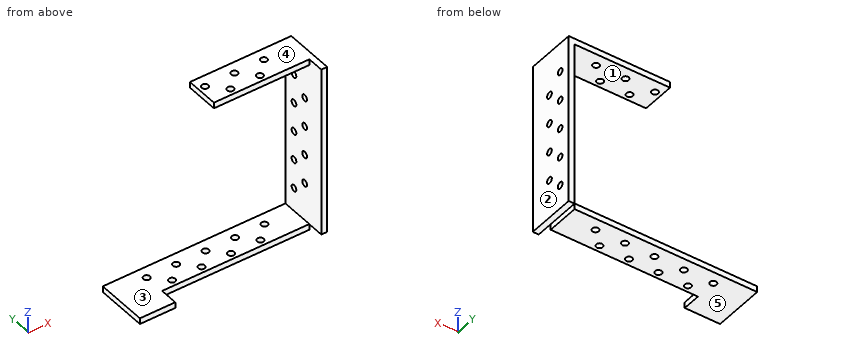
```python
from build123d import *

# Parameters (mm, degrees)
SKETCH1_W                      = 42
SKETCH1_H                      = 145.161285219
BOSS_EXTRUDE1_DEPTH            = 5
BOSS_EXTRUDE2_DEPTH            = 5
SKETCH3_W                      = 5
SKETCH3_H                      = 27.999999523
BOSS_EXTRUDE3_DEPTH            = 81.000003815
F_5_5_5_5_DIAMETER_HOLE1_D     = 5.5
F_5_5_5_5_DIAMETER_HOLE2_D     = 5.5
F_5_5_5_5_DIAMETER_HOLE2_DEPTH = 5
F_5_5_5_5_DIAMETER_HOLE3_D     = 5.5
F_5_5_5_5_DIAMETER_HOLE3_DEPTH = 5


with BuildPart() as part:
    # Sketch1 → Boss-Extrude1 (new body)
    with BuildSketch(Plane(origin=(-5, 0, 0), x_dir=(0, -1, 0), z_dir=(-1, 0, 0))):
        with Locations((21, -72.58064261)):
            Rectangle(SKETCH1_W, SKETCH1_H)
    extrude(amount=-BOSS_EXTRUDE1_DEPTH)

    # Sketch2 → Boss-Extrude2 (add)
    with BuildSketch(Plane(origin=(0, 0, -150), x_dir=(-1, 0, 0), z_dir=(0, 0, -1))):
        Polygon((130, -43.400001526), (160, -43.400001526), (160, 0), (5, 0), (5, -27.999999523), (130, -27.999999523), align=None)
    extrude(amount=-BOSS_EXTRUDE2_DEPTH)

    # Sketch3 → Boss-Extrude3 (add)
    with BuildSketch(Plane.ZY.offset(5)):
        with Locations((-2.5, -13.999999762)):
            Rectangle(SKETCH3_W, SKETCH3_H)
    extrude(amount=BOSS_EXTRUDE3_DEPTH)

    # Ø5.5 (5.5) Diameter Hole1 (through all)
    with Locations(Plane.ZY.offset(5)):
        with Locations((-37.500000596, -22.500000199), (-25.000000199, -9.99999995), (-50.000000795, -9.99999995), (-62.500000795, -22.500000199), (-75.000000795, -9.99999995), (-87.500000795, -22.500000199), (-112.500000795, -22.500000199), (-100.000000795, -9.99999995), (-125.000000795, -9.99999995)):
            Hole(F_5_5_5_5_DIAMETER_HOLE1_D / 2)

    # Ø5.5 (5.5) Diameter Hole2
    with Locations(Plane.XY.offset(-145)):
        with Locations((-30.000000199, -9.99999995), (-42.500000397, -22.500000199), (-67.500000795, -22.500000199), (-55.000000795, -9.99999995), (-80.000001192, -9.99999995), (-92.500000795, -22.500000199), (-117.500000795, -22.500000199), (-105.000000795, -9.99999995), (-130.000003179, -9.99999995)):
            Hole(F_5_5_5_5_DIAMETER_HOLE2_D / 2, depth=F_5_5_5_5_DIAMETER_HOLE2_DEPTH)

    # Ø5.5 (5.5) Diameter Hole3
    with Locations(Plane(origin=(0, 0, -5), x_dir=(-1, 0, 0), z_dir=(0, 0, -1))):
        with Locations((80.50000151, -9.99999995), (68.000001113, -22.500000199), (43.000001113, -22.500000199), (55.500001113, -9.99999995), (30.500000119, -9.99999995)):
            Hole(F_5_5_5_5_DIAMETER_HOLE3_D / 2, depth=F_5_5_5_5_DIAMETER_HOLE3_DEPTH)


solid = part.part
```
Build history of the part. All positions in model axes, mm. Face numbers are marked on the shaded views. A direction names the side the tool comes from. Round coordinates to 2 decimals unless told otherwise and drop trailing zeros. Order: outer loops, then holes, each group sorted by start corner. A loop starts at its lowest first (then second) coordinate and runs counter-clockwise, first axis right, second up. Notation, with made-up numbers: (10.25, -38) -> (19.25, -38) arc R3 cw to (19.25, -34) -> close; hole circle Ø6 at (35, 68). An arc over 180 degrees is marked (long way). Answer in a Markdown table with one row per item.
1) Pin check, flat tips, straight feed: P1, Ø4, axis at y = -8, z = -21, coming from the +X side; P2, Ø2.5, axis at y = -8.5, z = -2.5, coming from the -X side; P3, Ø5, axis at x = -30, y = -10, coming from the -Z side; P4, Ø5, axis at x = -92.5, y = -22.5, coming from the +Z side. Stop position of each tip, or through.
Values:
| item | result |
|---|---|
| P1 | x = 0 |
| P2 | x = -86 |
| P3 | z = -5 |
| P4 | through |
2) Band-saw the part on C-C on x = -67.5. Give the cut face in (y, z), and give its area (3 significant figures).
Values:
| item | result |
|---|---|
| outline | (-28, -150) -> (-25.25, -150) -> (-25.25, -145) -> (-28, -145) -> close; (-28, -5) -> (-25.2, -5) -> (-25.2, 0) -> (-28, 0) -> close; (-19.8, -5) -> (0, -5) -> (0, 0) -> (-19.8, 0) -> close; (-19.75, -150) -> (0, -150) -> (0, -145) -> (-19.75, -145) -> close |
| area | 225 mm2 |
3) Mould opens along Z. For the marked faces 3, 4 and 5 say: released by +Z, released by -Z, zero draft, split by the parting line, or undercut.
Values:
| item | result |
|---|---|
| face 3 | undercut |
| face 4 | released by +Z |
| face 5 | released by -Z |
4) Band-saw the part on D-D on x = -147.5. Give the cut face in (y, z).
Values:
| item | result |
|---|---|
| outline | (-43.4, -150) -> (0, -150) -> (0, -145) -> (-43.4, -145) -> close |
5) Which spindle directions (+Z, -Z, +X, -X, +Y, -Y) get a long thin tool onto all of the face, cutting with end or side? Do the marked faces 1 and 2. Say none if no direction does.
Values:
| item | result |
|---|---|
| face 1 | -X, +Y, -Y |
| face 2 | +Z, -Z, +X, +Y, -Y |
6) Wall check: L1, parallel to X at y = -22.5, z = -148.4; L2, parallel to X at y = -22, z = -146; L3, parallel to Z at x = -55.5, y = -6.5. Give the ranges that are in metal, low to high.
Values:
| item | result |
|---|---|
| L1 | -160 to -120.25, -114.75 to -95.25, -89.75 to -70.25, -64.75 to -45.25, -39.75 to -5 |
| L2 | -160 to -120.2, -114.8 to -95.2, -89.8 to -70.2, -64.8 to -45.2, -39.8 to -5 |
| L3 | -150 to -145, -5 to 0 |
7) Band-saw the part on A-A on z = -62.5. Give the cut face in (x, y), and give its area (4 significant figures).
Values:
| item | result |
|---|---|
| outline | (-5, -42) -> (0, -42) -> (0, -25.25) -> (-5, -25.25) -> close; (-5, -19.75) -> (0, -19.75) -> (0, 0) -> (-5, 0) -> close |
| area | 182.5 mm2 |
8) Band-saw the part on B-B on x = -117.5. Give the cut face in (y, z), and give its area (4 significant figures).
Values:
| item | result |
|---|---|
| outline | (-28, -150) -> (-25.25, -150) -> (-25.25, -145) -> (-28, -145) -> close; (-19.75, -150) -> (0, -150) -> (0, -145) -> (-19.75, -145) -> close |
| area | 112.5 mm2 |
